Source: three-view drawing plus pictorial views. Frame: mm from the lowest corner of the part. A direction names the side the tool comes from. Coordinates: 2 decimals unless noted, no trailing zeros. Write each loop counter-clockwise with the first axis right and the second up, starting at its lowest first coordinate (ties: lowest second). Pieces come first, ordered by that corner, then holes. Notation, with made-up numbers: (3, 60.5) - (11, 60.5) arc R14 ccw to (11, 87.5) - close; hole circle Ø8 at (43, 77.25). An arc over 180 degrees is marked (long way). One line per item, written item: value.
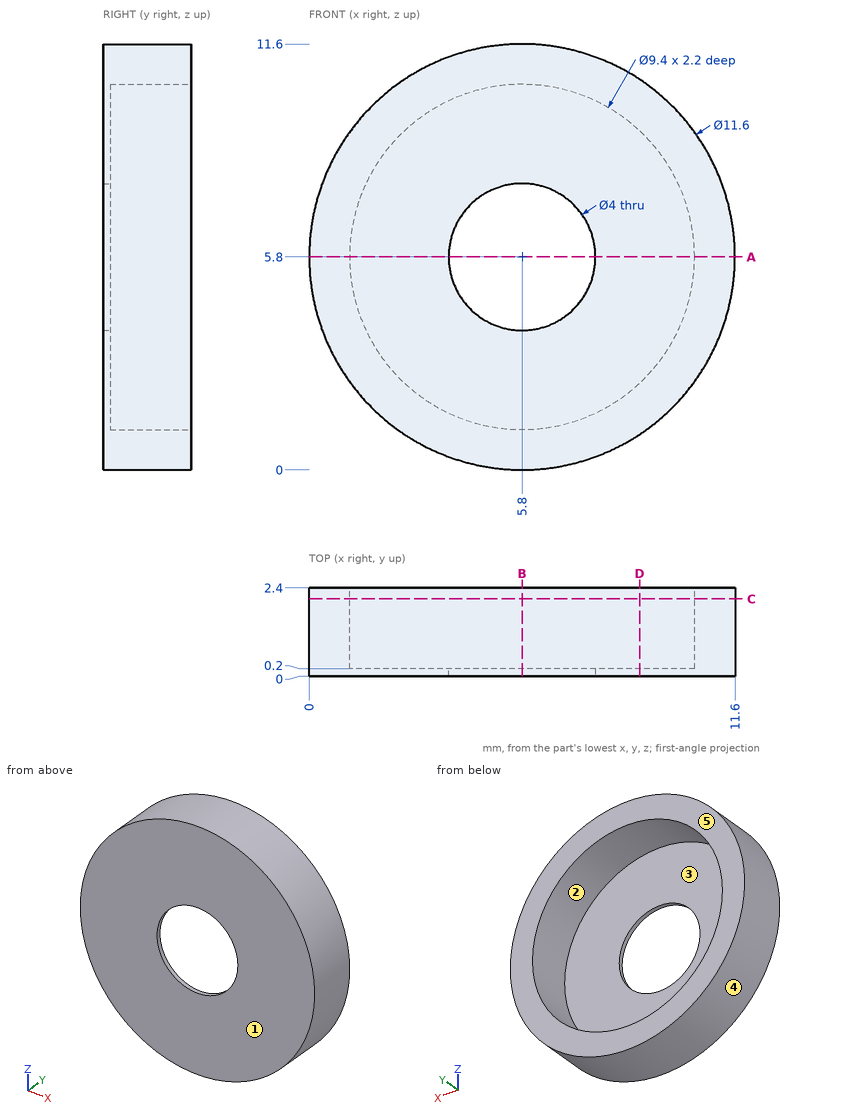
1) Draft query along Z for the marked faces 3, 4 and 5. Return one class per face: released by +Z, released by -Z, zero draft, split by the parting line, or undercut.
Values found:
face 3: undercut
face 4: split by the parting line
face 5: zero draft
2) Section query C-C on y = 2.1. Output: boundary loops of the cut face in (x, z), then the cut area to 3 significant figures.
Values found:
outline: circle Ø11.6 at (5.8, 5.8); hole circle Ø9.4 at (5.8, 5.8)
area: 36.3 mm2
3) Section query A-A on z = 5.8. Output: boundary loops of the cut face in (x, y).
Values found:
outline: (0, 0) - (3.8, 0) - (3.8, 0.2) - (1.1, 0.2) - (1.1, 2.4) - (0, 2.4) - close; (7.8, 0) - (11.6, 0) - (11.6, 2.4) - (10.5, 2.4) - (10.5, 0.2) - (7.8, 0.2) - close
4) Material intervals for line 1 (Z direction, x = 5.8, y = 0.15); line 2 (X direction, y = 0.55, z = 5.75), sorted ascending.
Values found:
line 1: 0 to 3.8, 7.8 to 11.6
line 2: 0 to 1.1, 10.5 to 11.6
5) Section query B-B on x = 5.8. Output: boundary loops of the cut face in (y, z), then the cut area to 3 significant figures.
Values found:
outline: (0, 0) - (2.4, 0) - (2.4, 1.1) - (0.2, 1.1) - (0.2, 3.8) - (0, 3.8) - close; (0, 7.8) - (0.2, 7.8) - (0.2, 10.5) - (2.4, 10.5) - (2.4, 11.6) - (0, 11.6) - close
area: 6.36 mm2
6) Contact query for a flat-ended pin moving along its axis: P1, Ø1, axis at x = 9, y = 0.5, coming from the -Z side. Output: stop coordinate, or through.
Values found:
P1: z = 0.67
7) Reachability of the marked faces 1 and 2 from +Z, -Z, +X, -X, +Y, -Y: full face, straight path, thin tool, end or side. Return the list, or none.
Values found:
face 1: +Z, -Z, +X, -X, -Y
face 2: +Y
8) Section query D-D on x = 9. Output: boundary loops of the cut face in (y, z), then the cut area to 3 significant figures.
Values found:
outline: (0, 0.96) - (2.4, 0.96) - (2.4, 2.36) - (0.2, 2.36) - (0.2, 9.24) - (2.4, 9.24) - (2.4, 10.64) - (0, 10.64) - close
area: 8.07 mm2
